Source: CAD feature listing. Evaluate the final solid. Frame: model axes, mm. A direction names the side the tool comes from. Give positions to 0.01 mm unless a question says otherwise; leave off trailing zeros. Order: outer loops, then holes, each group sorted by start corner. A loop starts at its lowest first (then second) coordinate and runs counter-clockwise, first axis right, second up. Notation, with made-up numbers: (2.5, 77) - (33.5, 77) arc R32 cw to (33.5, 114) - close; hole circle Ø8 at (86, 39). An arc over 180 degrees is marked (long way). Write each question's results on one line, items separated by ' | '. Start each with the question number.
Item 1: Section C-C on y = 3. Output: boundary loops of the cut face in (x, z).
Item 2: Line query: line 1 along Y through (x, z) = (-1.75, 0.8); line 2 along Z through (x, y) = (-0.5, -3.25). Output: solid intervals per line, ascending.
Item 3: Section B-B on y = 2. Output: boundary loops of the cut face in (x, z), and give its area (3 significant figures).
Item 4: Set-up query: faces 1 (the cylindrical face through (-3.34, -1.57, 0.59)), 2 (the flat face through (-1, -3, 1.2)), 3 (the cylindrical face through (-3.3, 1.61, 0.59)). Return all of +Z, -Z, +X, -X, +Y, -Y with unobstructed straight access to the full face (end or side cutting, diameter ignored); none if empty.
Item 5: Section A-A on z = 1.55. Output: boundary loops of the cut face in (x, y).
Item 6: Contact query for flat-ended pins moving along their axis: pin 1 Ø2 at (x, z) = (10, 1.5) entering from -Y; pin 2 Ø0.6 at (x, z) = (1.5, 1) entering from +Y; pin 3 Ø1 at (x, z) = (3, 0.5) entering from -Y. Output: stop coordinate, or through.
```python
from build123d import *

# Parameters (mm, degrees)
F6_W      = 19.1
F6_H      = 8.9
F7_DEPTH  = 1.2
F10_DEPTH = 1.2
F11_R     = 2.24999
F12_W     = 19.1
F12_H     = 8.9
F13_DEPTH = 4.2
F14_DEPTH = 4
F15_W     = 19.1
F15_H     = 8.9
F16_DEPTH = 5.2


# Not quite as in the source:
# - a fillet or chamfer is up to 0.001 mm smaller than in the source, because OpenCascade refuses the exact size


with BuildPart() as f7:
    # F6 (on Top) → F7 (new body, through all)
    with BuildSketch(Plane.XY):
        with Locations((3.24578159, 0)):
            Rectangle(F6_W, F6_H)
    extrude(amount=F7_DEPTH)

    # F8 (on face) → F10 (cut, through all)
    with BuildSketch(Plane.XY.offset(1.2)):
        with BuildLine():
            Line((4.7402303145, 2.25), (-3.97921841, 2.25))
            Line((-3.97921841, 2.25), (-3.97921841, -2.25))
            Line((-3.97921841, -2.25), (4.7402303145, -2.25))
            ThreePointArc((4.7402303145, -2.25), (4.09578159, 0), (4.7402303145, 2.25))
        make_face()
        with BuildLine():
            ThreePointArc((12.59578159, 0), (9.5160181215, 4.0857124789), (4.7402303145, 2.25))
            ThreePointArc((4.7402303145, 2.25), (4.09578159, 0), (4.7402303145, -2.25))
            ThreePointArc((4.7402303145, -2.25), (9.5160181215, -4.0857124789), (12.59578159, 0))
        make_face()
    extrude(amount=-F10_DEPTH, mode=Mode.SUBTRACT)

    # F11 (radius 2.25 in the source; OpenCascade refuses exactly that, so slightly less here)
    f11_edges = [f7.edges().sort_by_distance(p)[0] for p in [
        (-3.979218, 2.25, 0.6),
        (-3.979218, -2.25, 0.6),
    ]]
    fillet(f11_edges, radius=F11_R)

    # F12 (on face) → F13 (join)
    with BuildSketch(Plane.XY.offset(1.2)):
        with Locations((3.24578159, 0)):
            Rectangle(F12_W, F12_H)
    extrude(amount=F13_DEPTH)

    # F9 (on offset) → F14 (cut, through all)
    with BuildSketch(Plane.XY.offset(1.2)):
        with BuildLine():
            Line((-1.85421841, -4.25), (8.34578159, -4.25))
            ThreePointArc((8.34578159, -4.25), (12.59578159, 0), (8.34578159, 4.25))
            Line((8.34578159, 4.25), (-1.85421841, 4.25))
            ThreePointArc((-1.85421841, 4.25), (1.15098541, 3.00520382), (2.39578159, 0))
            ThreePointArc((2.39578159, 0), (1.15098541, -3.00520382), (-1.85421841, -4.25))
        make_face()
        with BuildLine():
            ThreePointArc((-1.85421841, 4.25), (-6.10421841, 0), (-1.85421841, -4.25))
            ThreePointArc((-1.85421841, -4.25), (1.15098541, -3.00520382), (2.39578159, 0))
            ThreePointArc((2.39578159, 0), (1.15098541, 3.00520382), (-1.85421841, 4.25))
        make_face()
    extrude(amount=F14_DEPTH, mode=Mode.SUBTRACT)


with BuildPart() as f16:
    # F15 (on face) → F16 (new body, through all)
    with BuildSketch(Plane(origin=(0, 0, 0), x_dir=(1, 0, 0), z_dir=(0, 0, -1))):
        with Locations((3.24578159, 0)):
            Rectangle(F15_W, F15_H)
    extrude(amount=-F16_DEPTH)

    # F17: cut F7
    add(f7.part, mode=Mode.SUBTRACT)


solid = f16.part
```
Evaluation:
1) outline: (-4.86, 1.2) - (5.34, 1.2) - (5.34, 0) - (11.36, 0) - (11.36, 5.2) - (-4.86, 5.2) - close
2) line 1: y = -2.25 to 2.25 | line 2: z = 1.2 to 5.2
3) outline: (-5.6, 1.2) - (-2.76, 1.2) - (-2.76, 0) - (12.1, 0) - (12.1, 5.2) - (-5.6, 5.2) - close | area: 88.6 mm^2
4) face 1: -Z, -X, -Y | face 2: -Z, -X, -Y | face 3: -Z, -X, +Y
5) outline: (-1.85, -4.25) - (8.35, -4.25) arc R4.25 ccw to (8.35, 4.25) - (-1.85, 4.25) arc R4.25 ccw to start
6) pin 1: stops at y = -4.2 | pin 2: stops at y = 4.25 | pin 3: stops at y = -2.25
